from build123d import *

# Parameters (mm, degrees)
F0_W     = 450
F0_H     = 450
F1_DEPTH = 950
F2_W     = 50
F2_H     = 409.0744554996
F2_W_2   = 335
F2_H_2   = 50
F3_DEPTH = 450.001
F4_W     = 380
F4_H     = 409.074
F5_DEPTH = 450.001
F6_W     = 380
F6_H     = 50
F6_H_2   = 318.4651864549
F7_DEPTH = 126.1046604873


with BuildPart() as f1:
    # F0 (on Top) → F1 (new body)
    with BuildSketch(Plane.XY):
        Rectangle(F0_W, F0_H)
    extrude(amount=F1_DEPTH)

    # F2 (on face) → F3 (cut, through all)
    with BuildSketch(Plane.YZ.offset(225)):
        Polygon((225, 950), (175, 459.0744554996), (225, 459.0744554996), align=None)
        Polygon((-225, 950), (-225, 459.0744554996), (145, 459.0744554996), (195, 950), align=None)
        with Locations((200, 204.5372277498)):
            Rectangle(F2_W, F2_H)
        with Locations((-22.5, 204.5372277498)):
            Rectangle(F2_W_2, F2_H)
        with Locations((200, 434.0744554996)):
            Rectangle(F2_W, F2_H_2)
    extrude(amount=-F3_DEPTH, mode=Mode.SUBTRACT)

    # F4 (on face) → F5 (cut, through all)
    with BuildSketch(Plane.XZ.offset(225)):
        with Locations((0, 204.537)):
            Rectangle(F4_W, F4_H)
    extrude(amount=-F5_DEPTH, mode=Mode.SUBTRACT)

    # F6 (on face) → F7 (cut, through all)
    with BuildSketch(Plane(origin=(0, 97.2353512241, -9.903268664), x_dir=(1, 0, 0), z_dir=(0, -0.9948534526, 0.1013242704))):
        with Locations((0, 864.869012738)):
            Rectangle(F6_W, F6_H)
        with Locations((0, 630.6364195106)):
            Rectangle(F6_W, F6_H_2)
    extrude(amount=-F7_DEPTH, mode=Mode.SUBTRACT)


solid = f1.part
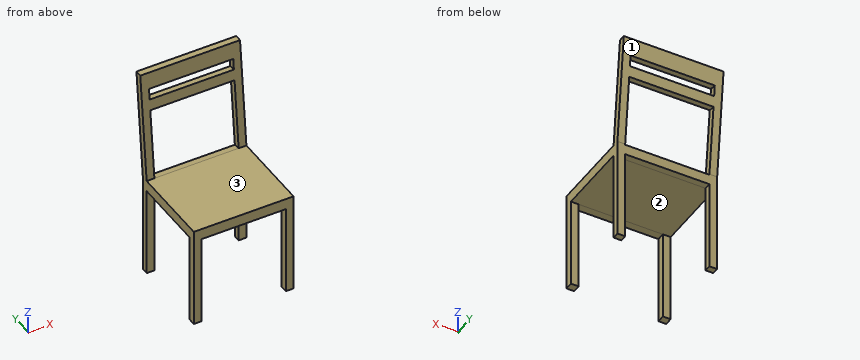
The model under review builds one solid part; all positions refer to its coordinate system, in mm. Face numbers are marked on the shaded views. A direction names the side the tool comes from. Round coordinates to 2 decimals unless told otherwise and drop trailing zeros. Loops run counter-clockwise (first coordinate to the right, second up) from the corner with the lowest first, then second, coordinate; pieces in that order, holes last. Notation, with made-up numbers: (33, 62) -> (73, 62) arc R11 cw to (73, 66) -> close; hole circle Ø5 at (-35, 54.25). An arc over 180 degrees is marked (long way). Return JSON: item names as keys, results as strings.
(1) Add section C-C on z = 658. Write out the cut boundary in (x, y).
Solved:
{"outline": "(-225, 165.26) -> (-190, 165.26) -> (-190, 195.26) -> (-225, 195.26) -> close; (190, 165.26) -> (225, 165.26) -> (225, 195.26) -> (190, 195.26) -> close"}
(2) For pin 1 (4 mm diameter, centred on x = -163, z = 812.5, fed in from +Y); pin 2 (8 mm diameter, centred on x = 30, y = 4.5, fed in from -Z); pin 3 (10 mm diameter, centred on x = 30, y = 56, fed in from +Z), all flat-tipped, find the tip position at first contact; note any pin that passes through.
Solved:
{"pin 1": "y = 211.2", "pin 2": "z = 409.07", "pin 3": "z = 459.07"}
(3) Add section A-A on z = 303. Write out the cut boundary in (x, y), plus the area to 3 significant figures.
Solved:
{"outline": "(-225, -225) -> (-190, -225) -> (-190, -190) -> (-225, -190) -> close; (-225, 145) -> (-190, 145) -> (-190, 175) -> (-225, 175) -> close; (190, -225) -> (225, -225) -> (225, -190) -> (190, -190) -> close; (190, 145) -> (225, 145) -> (225, 175) -> (190, 175) -> close", "area": "4,550 mm2"}
(4) Add section B-B on x = 26. State how many separate pieces and enclosed holes the cut face has, plus the area to 3 significant figures.
Solved:
{"separate pieces": "3", "enclosed holes": "0", "area": "23,700 mm2"}
(5) For line 1 (Z direction, x = -125, y = -100.5); line 2 (Y direction, x = 202.5, z = 417); line 3 (Y direction, x = 43.5, z = 801), list the stretches that pass through material, from the lowest coordinate up.
Solved:
{"line 1": "409.07 to 459.07", "line 2": "-225 to 175", "line 3": "179.82 to 209.82"}
(6) For the marked faces 1, 2 and 3, list the 3-axis set-ups (+Z, -Z, +X, -X, +Y, -Y) from which the entire face can be reached by the end or side of a thin tool; tool diameter is ignored.
Solved:
{"face 1": "-Z, +X, -X, +Y", "face 2": "-Z, +X, -X", "face 3": "+Z, +X, -X, -Y"}
(7) Add section D-D on y = 156. Write out the cut boundary in (x, z), plus the area to 3 significant figures.
Solved:
{"outline": "(-225, 0) -> (-190, 0) -> (-190, 409.07) -> (190, 409.07) -> (190, 0) -> (225, 0) -> (225, 567.08) -> (190, 567.08) -> (190, 457.95) -> (-190, 457.95) -> (-190, 567.08) -> (-225, 567.08) -> close", "area": "58,300 mm2"}
